Input: part model. Units: mm. Frame: model coordinates. A direction names the side the tool comes from. Round coordinates to 2 decimals unless told otherwise and drop trailing zeros. Order: outer loops, then holes, each group sorted by start corner. A loop starts at its lowest first (then second) coordinate and runs counter-clockwise, first axis right, second up. Notation, with made-up numbers: (45, 61) -> (84, 61) arc R33 cw to (84, 93) -> close; hole circle Ø11 at (12, 8.5). An arc over 180 degrees is marked (long way). Use a Markdown table: item, result.
from build123d import *

# Parameters (mm, degrees)
SKETCH1_R           = 3
SKETCH1_R_2         = 2
BOSS_EXTRUDE1_DEPTH = 10
BOSS_EXTRUDE2_DEPTH = 2
BOSS_EXTRUDE3_DEPTH = 10


with BuildPart() as part:
    # Sketch1 → Boss-Extrude1 (new body)
    with BuildSketch(Plane.XY):
        Circle(SKETCH1_R)
        Circle(SKETCH1_R_2, mode=Mode.SUBTRACT)
    extrude(amount=BOSS_EXTRUDE1_DEPTH)

    # Sketch2 → Boss-Extrude2 (add)
    with BuildSketch(Plane(origin=(0, 0, 0), x_dir=(-1, 0, 0), z_dir=(0, 0, -1))):
        Polygon((0, -5), (15, -5), (15, 5), (-15, 5), (-15, -5), align=None)
    extrude(amount=BOSS_EXTRUDE2_DEPTH)

    # Sketch3 → Boss-Extrude3 (add)
    with BuildSketch(Plane(origin=(0, 5, 0), x_dir=(1, 0, 0), z_dir=(0, 1, 0))):
        Polygon((-0.707106781, 1.292893219), (0, 2), (0.707106781, 1.292893219), (14.849242405, 15.435028843), (13.435028843, 16.849242405), (0, 3.414213562), (-13.435028843, 16.849242405), (-14.849242405, 15.435028843), align=None)
    extrude(amount=-BOSS_EXTRUDE3_DEPTH)


solid = part.part
1) Cut plane A-A on z = -10.5. Return loops of the section in (x, y), and give its area (3 significant figures).
Answer key:
| item | result |
|---|---|
| outline | (-9.91, -5) -> (-7.09, -5) -> (-7.09, 5) -> (-9.91, 5) -> close; (7.09, -5) -> (9.91, -5) -> (9.91, 5) -> (7.09, 5) -> close |
| area | 56.6 mm^2 |
2) Set-up query: faces 1 (the face through (0, -2, 5)), 2 (the face through (-2, -5, -5)), 3 (the face through (-8.226, 0.07, -8.812)), 4 (the face through (8, 0, -2)), 5 (the face through (6.812, 0.07, -10.226)). Return all of +Z, -Z, +X, -X, +Y, -Y with unobstructed straight access to the full face (end or side cutting, diameter ignored); none if empty.
Answer key:
| item | result |
|---|---|
| face 1 | +Z |
| face 2 | +Z, -Z, +X, -X, -Y |
| face 3 | -X, +Y, -Y |
| face 4 | +X, +Y, -Y |
| face 5 | -Z, +Y, -Y |
3) Cut plane C-C on x = 8. Return loops of the section in (y, z), and give its area (3 significant figures).
Answer key:
| item | result |
|---|---|
| outline | (-5, -11.41) -> (5, -11.41) -> (5, -8.59) -> (-5, -8.59) -> close; (-5, -2) -> (5, -2) -> (5, 0) -> (-5, 0) -> close |
| area | 48.3 mm^2 |
4) Ray query, probe 1 along Y at (x, z) = (0, 8.25); probe 2 along Z at (x, y) = (4.25, 0.5); probe 3 along Z at (x, y) = (-11.25, 2.75). Return the intervals inside material, ascending.
Answer key:
| item | result |
|---|---|
| probe 1 | y = -3 to -2, 2 to 3 |
| probe 2 | z = -7.66 to -4.84, -2 to 0 |
| probe 3 | z = -14.66 to -11.84, -2 to 0 |
5) Contact query for flat-ended pins moving along their axis: P1, Ø3, axis at x = -11, y = 1, coming from the -Z side; P2, Ø5, axis at x = 7, y = -2, coming from the +Z side; P3, Ø3, axis at x = 7.5, y = -3, coming from the -Z side. Output: stop coordinate, or through.
Answer key:
| item | result |
|---|---|
| P1 | stops at z = -15.91 |
| P2 | stops at z = 0 |
| P3 | stops at z = -12.41 |
6) Cut plane B-B on y = 4.25. Return loops of the section in (x, z).
Answer key:
| item | result |
|---|---|
| outline | (-15, -2) -> (-1.41, -2) -> (-14.85, -15.44) -> (-13.44, -16.85) -> (0, -3.41) -> (13.44, -16.85) -> (14.85, -15.44) -> (1.41, -2) -> (15, -2) -> (15, 0) -> (-15, 0) -> close |
7) Cut plane D-D on z = 2.5. Return loops of the section in (x, y).
Answer key:
| item | result |
|---|---|
| outline | circle Ø6 at (0, 0); hole circle Ø4 at (0, 0) |
8) Draft query along Z for faces 6 (the face through (8.038, 0.07, -8.623)), 7 (the face through (-15, 0, -1)), 8 (the face through (-8, 0, -2)), 9 (the face through (-6.623, 0.07, -10.038)). Return one class per face: released by +Z, released by -Z, zero draft, split by the parting line, or undercut.
Answer key:
| item | result |
|---|---|
| face 6 | undercut |
| face 7 | zero draft |
| face 8 | undercut |
| face 9 | released by -Z |
